Part model, mm, in its own coordinate system. Coordinates: 2 decimals unless noted, no trailing zeros. Loops run counter-clockwise (first coordinate to the right, second up) from the corner with the lowest first, then second, coordinate; pieces in that order, holes last.
```python
from build123d import *

# Parameters (mm, degrees)
F0_W     = 86.138785
F0_H     = 46.305328
F1_DEPTH = 25.4
F3_DEPTH = 48.26
F5_DEPTH = 50.8


with BuildPart() as f1:
    # F0 (on Front) → F1 (new body)
    with BuildSketch(Plane.XZ):
        with Locations((1.097095, -11.160776)):
            Rectangle(F0_W, F0_H)
    extrude(amount=F1_DEPTH)

    # F2 (on face) → F3 (cut)
    with BuildSketch(Plane(origin=(0, 0, -34.31344), x_dir=(1, 0, 0), z_dir=(0, 0, -1))):
        Polygon((-41.972298, 12.7), (-10.236957, 25.4), (-41.972298, 25.4), align=None)
    extrude(amount=-F3_DEPTH, mode=Mode.SUBTRACT)

    # F4 (on face) → F5 (cut)
    with BuildSketch(Plane(origin=(0, 0, -34.31344), x_dir=(1, 0, 0), z_dir=(0, 0, -1))):
        Polygon((-41.972298, 0), (-10.572781, 0), (-41.972298, 8.64746), align=None)
    extrude(amount=-F5_DEPTH, mode=Mode.SUBTRACT)


solid = f1.part
```
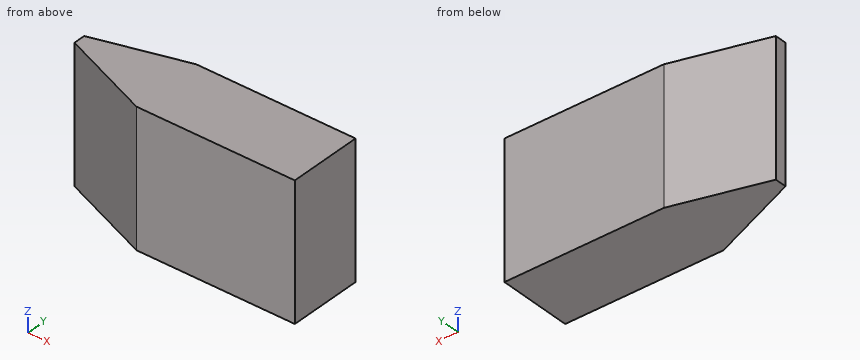
Q1. Drop flat-ended pins along their axis: P1, Ø12, axis at x = -28.5, z = -5, coming from the +Y side; P2, Ø6, axis at y = -16.5, z = -19, coming from the -X side; P3, Ø5, axis at x = -19.5, z = -21.5, coming from the -Y side. Give the stop position or say it passes through.
Q2. Saw through at A-A (z = -10). List the corners of the cut face in (x, y).
Q3. Saw through at B-B (y = -16). List the corners of the cut face in (x, z), plus the area to 3 significant figures.
Q4. Probe line 1 (X direction, y = -21.25, z = 8.5); line 2 (Y direction, x = -18, z = 2.5); line 3 (Y direction, x = -23.5, z = -5). List the from-to ranges inside material, lowest first.
Q5. Saw through at C-C (x = -30). List the corners of the cut face in (y, z).
Checked values:
1. P1: stops at y = -3.28
1. P2: stops at x = -39.97
1. P3: stops at y = -22.69
2. outline: (-41.97, -12.7) - (-10.24, -25.4) - (44.17, -25.4) - (44.17, 0) - (-10.57, 0) - (-41.97, -8.65) - close
3. outline: (-33.73, -34.31) - (44.17, -34.31) - (44.17, 11.99) - (-33.73, 11.99) - close
3. area: 3,610 mm2
4. line 1: x = -20.61 to 44.17
4. line 2: y = -22.29 to -2.05
4. line 3: y = -20.09 to -3.56
5. outline: (-17.49, -34.31) - (-5.35, -34.31) - (-5.35, 11.99) - (-17.49, 11.99) - close
